CAD build for the part. Positions are in the model's coordinates, mm. A direction names the side the tool comes from. Round coordinates to 2 decimals unless told otherwise and drop trailing zeros. Loops run counter-clockwise (first coordinate to the right, second up) from the corner with the lowest first, then second, coordinate; pieces in that order, holes last.
```python
from build123d import *

# Parameters (mm, degrees)
SKETCH1_R           = 20
BOSS_EXTRUDE1_DEPTH = 15
SKETCH2_R           = 12.5
CUT_EXTRUDE1_DEPTH  = 10
SKETCH3_R           = 6
CUT_EXTRUDE2_DEPTH  = 5
SKETCH4_R           = 1.5
CUT_EXTRUDE3_DEPTH  = 15
SKETCH5_R           = 1.5
CUT_EXTRUDE4_DEPTH  = 5


with BuildPart() as part:
    # Sketch1 → Boss-Extrude1 (new body)
    with BuildSketch(Plane(origin=(0, 0, 0), x_dir=(1, 0, 0), z_dir=(0, 1, 0))):
        Circle(SKETCH1_R)
    extrude(amount=BOSS_EXTRUDE1_DEPTH)

    # Sketch2 → Cut-Extrude1 (cut)
    with BuildSketch(Plane(origin=(0, 15, 0), x_dir=(1, 0, 0), z_dir=(0, 1, 0))):
        Circle(SKETCH2_R)
    extrude(amount=-CUT_EXTRUDE1_DEPTH, mode=Mode.SUBTRACT)

    # Sketch3 → Cut-Extrude2 (cut)
    with BuildSketch(Plane(origin=(0, 5, 0), x_dir=(1, 0, 0), z_dir=(0, 1, 0))):
        Circle(SKETCH3_R)
    extrude(amount=-CUT_EXTRUDE2_DEPTH, mode=Mode.SUBTRACT)

    # Sketch4 → Cut-Extrude3 (cut)
    with BuildSketch(Plane(origin=(0, 15, 0), x_dir=(1, 0, 0), z_dir=(0, 1, 0))):
        with Locations((-10.493132047, -12.733584721)):
            Circle(SKETCH4_R)
        with Locations((-16.274173873, 2.720526557)):
            Circle(SKETCH4_R)
        with Locations((-5.781041827, 15.454111278)):
            Circle(SKETCH4_R)
        with Locations((10.493132047, 12.733584721)):
            Circle(SKETCH4_R)
        with Locations((16.274173873, -2.720526557)):
            Circle(SKETCH4_R)
        with Locations((5.781041827, -15.454111278)):
            Circle(SKETCH4_R)
    extrude(amount=-CUT_EXTRUDE3_DEPTH, mode=Mode.SUBTRACT)

    # Sketch5 → Cut-Extrude4 (cut)
    with BuildSketch(Plane.XZ):
        with Locations((0, 8.5)):
            Circle(SKETCH5_R)
        with Locations((0, -8.5)):
            Circle(SKETCH5_R)
    extrude(amount=-CUT_EXTRUDE4_DEPTH, mode=Mode.SUBTRACT)


solid = part.part
```
Item 1: Probe line 1 (Y direction, x = 11, z = -1.5); line 2 (Z direction, x = 0.5, y = 3.5); line 3 (Z direction, x = 6.5, y = 10.5). List the from-to ranges inside material, lowest first.
Answers follow:
line 1: y = 0 to 5
line 2: z = -19.99 to -9.91, -7.09 to -5.98, 5.98 to 7.09, 9.91 to 19.99
line 3: z = -18.91 to -10.68, 10.68 to 14.14, 16.77 to 18.91
Item 2: 3-axis set-ups, long thin cutter, end or side, ignore diameter. For faces 1 (the cylindrical face through (11.3, 7.6, -14)), 2 (the cylindrical face through (11.923, 10.07, -3.755)): which of +Z, -Z, +X, -X, +Y, -Y reach the whole face in a straight line?
Answers follow:
face 1: +Y, -Y
face 2: +Y
Item 3: Cut at A-A, the plane z = 0. Give the cut face in (x, y).
Answers follow:
outline: (-20, 0) - (-6, 0) - (-6, 5) - (-12.5, 5) - (-12.5, 15) - (-20, 15) - close; (6, 0) - (20, 0) - (20, 15) - (12.5, 15) - (12.5, 5) - (6, 5) - close
Item 4: Two-plate mould, pull along Z, no slides. Class faces 3 (the cylindrical face through (-4.336, 7.395, 19.524)), 4 (the flat face through (9, 15, -9)), 5 (the cylindrical face through (17.705, 7.605, 2.27)): released by +Z, released by -Z, zero draft, split by the parting line, or undercut.
Answers follow:
face 3: split by the parting line
face 4: zero draft
face 5: undercut
Item 5: Cut at C-C, the plane y = 2.75. State how many separate pieces and enclosed holes the cut face has, plus the area to 3 significant figures.
Answers follow:
separate pieces: 1
enclosed holes: 9
area: 1,090 mm2
Item 6: Cut at B-B, the plane x = 6.5. Give the cut face in (y, z).
Answers follow:
outline: (0, -18.91) - (15, -18.91) - (15, -10.68) - (5, -10.68) - (5, 10.68) - (15, 10.68) - (15, 14.14) - (0, 14.14) - close; (0, 16.77) - (15, 16.77) - (15, 18.91) - (0, 18.91) - close
Item 7: Flat gauge pins, fed straight in: P1, Ø2, axis at x = -2, z = 4, coming from the -Y side; P2, Ø1.5, axis at x = 14, y = 7.5, coming from the -Z side; P3, Ø8, axis at x = -4.5, z = -3.5, coming from the +Y side; P4, Ø2, axis at y = 4, z = -4, coming from the +X side. Where does each tip first touch, or does it go through?
Answers follow:
P1: passes through
P2: stops at z = -14.98
P3: stops at y = 5
P4: stops at x = 19.77
Item 8: Cut at D-D, the plane x = 0. Give the cut face in (y, z), plus the area to 3 significant figures.
Answers follow:
outline: (0, -20) - (15, -20) - (15, -12.5) - (5, -12.5) - (5, -10) - (0, -10) - close; (0, -7) - (5, -7) - (5, -6) - (0, -6) - close; (0, 6) - (5, 6) - (5, 7) - (0, 7) - close; (0, 10) - (5, 10) - (5, 12.5) - (15, 12.5) - (15, 20) - (0, 20) - close
area: 260 mm2
